```python
from build123d import *
from build123d import SkipClean  # not in build123d's __all__

# Parameters (mm, degrees)
F1_DEPTH  = 25.4
F1_FACE_R = 17.6985452631
F2_DEPTH  = 25.4
F3_DEPTH  = 25.4


with BuildPart() as f1:
    # F0 (on Top) → F1 (new body)
    with BuildSketch(Plane.XY):
        with BuildLine():
            ThreePointArc((0, 41.7947099158), (29.5533227992, 29.5533227992), (41.7947099158, 0))
            ThreePointArc((41.7947099158, 0), (29.5533227992, -29.5533227992), (0, -41.7947099158))
            Line((0, -41.7947099158), (0, -41.9407263398))
            Line((0, -41.9407263398), (115.8670112491, -41.9407263398))
            Line((115.8670112491, -41.9407263398), (115.8670112491, 41.7947099158))
            Line((115.8670112491, 41.7947099158), (0, 41.7947099158))
        make_face()
        with BuildLine():
            ThreePointArc((0, -41.7947099158), (29.5533227992, -29.5533227992), (41.7947099158, 0))
            ThreePointArc((41.7947099158, 0), (29.5533227992, 29.5533227992), (0, 41.7947099158))
            Line((0, 41.7947099158), (0, 17.6985452631))
            ThreePointArc((0, 17.6985452631), (12.5147613727, 12.5147613727), (17.6985452631, 0))
            ThreePointArc((17.6985452631, 0), (12.5147613727, -12.5147613727), (0, -17.6985452631))
            Line((0, -17.6985452631), (0, -41.7947099158))
        make_face()
        with BuildLine():
            Line((0, 17.6985452631), (0, 41.7947099158))
            ThreePointArc((0, 41.7947099158), (-41.7947099158, 0), (0, -41.7947099158))
            Line((0, -41.7947099158), (0, -17.6985452631))
            ThreePointArc((0, -17.6985452631), (-17.6985452631, 0), (0, 17.6985452631))
        make_face()
    extrude(amount=F1_DEPTH)

    # F1_face (on face) + F0 (on Top) → F2 (join)
    with BuildSketch(Plane(origin=(44.792448598, -0.0617990101, 25.4), x_dir=(1, 0, 0), z_dir=(0, 0, 1))):
        with BuildLine():
            Line((71.0745626511, 41.8565089259), (-44.792448598, 41.8565089259))
            ThreePointArc((-44.792448598, 41.8565089259), (-86.5871585138, 0.0617990101), (-44.792448598, -41.7329109057))
            Line((-44.792448598, -41.7329109057), (-44.792448598, -41.8789273297))
            Line((-44.792448598, -41.8789273297), (71.0745626511, -41.8789273297))
            Line((71.0745626511, -41.8789273297), (71.0745626511, 41.8565089259))
        make_face()
        with Locations((-44.792448598, 0.0617990101)):
            Circle(F1_FACE_R, mode=Mode.SUBTRACT)
    with BuildSketch(Plane.XY):
        with BuildLine():
            ThreePointArc((0, -41.7947099158), (29.5533227992, -29.5533227992), (41.7947099158, 0))
            ThreePointArc((41.7947099158, 0), (29.5533227992, 29.5533227992), (0, 41.7947099158))
            Line((0, 41.7947099158), (0, 17.6985452631))
            ThreePointArc((0, 17.6985452631), (12.5147613727, 12.5147613727), (17.6985452631, 0))
            ThreePointArc((17.6985452631, 0), (12.5147613727, -12.5147613727), (0, -17.6985452631))
            Line((0, -17.6985452631), (0, -41.7947099158))
        make_face()
        with BuildLine():
            ThreePointArc((0, 41.7947099158), (29.5533227992, 29.5533227992), (41.7947099158, 0))
            ThreePointArc((41.7947099158, 0), (29.5533227992, -29.5533227992), (0, -41.7947099158))
            Line((0, -41.7947099158), (0, -41.9407263398))
            Line((0, -41.9407263398), (115.8670112491, -41.9407263398))
            Line((115.8670112491, -41.9407263398), (115.8670112491, 41.7947099158))
            Line((115.8670112491, 41.7947099158), (0, 41.7947099158))
        make_face()
        with BuildLine():
            Line((0, 17.6985452631), (0, 41.7947099158))
            ThreePointArc((0, 41.7947099158), (-41.7947099158, 0), (0, -41.7947099158))
            Line((0, -41.7947099158), (0, -17.6985452631))
            ThreePointArc((0, -17.6985452631), (-17.6985452631, 0), (0, 17.6985452631))
        make_face()
    with SkipClean():  # cleaning this boolean's faces spoils the solid; the shape is the same uncleaned
        extrude(amount=F2_DEPTH)

    # F3 (cut): a face of the model
    f3_faces = [f1.faces().sort_by_distance(p)[0] for p in [
        (44.792448598, -0.0617990101, 50.8),
    ]]
    extrude(f3_faces, amount=-F3_DEPTH, mode=Mode.SUBTRACT)


solid = f1.part
```
Source: CAD feature listing. Evaluate the final solid. Frame: model axes, mm. Give positions to 0.01 mm unless a question says otherwise; leave off trailing zeros. Write each loop counter-clockwise with the first axis right and the second up, starting at its lowest first coordinate (ties: lowest second). Pieces come first, ordered by that corner, then holes.
1. Section query B-B (y = 7). Return the cut outline in (x, z), then the cut area to 3 significant figures.
2. First-contact query: pin 1 (2 mm diameter, centred on y = -3, z = 9, fed in from -X); pin 2 (10 mm diameter, centred on x = -20.5, z = 12.5, fed in from -Y); pin 3 (12 mm diameter, centred on x = -12, z = 20.5, fed in from +Y). Flat tips, straight axial feed; report the tip coordinate or a pass-through.
3. Section query C-C (y = 23.5). Return the cut outline in (x, z).
4. Section query A-A (z = 6.5). Return the cut outline in (x, y), then the cut area to 3 significant figures.
5. Section query D-D (y = -23). Return the cut outline in (x, z), then the cut area to 3 significant figures.
6. Material intervals for line 1 along Y through (x, z) = (1, 2.25); line 2 along Y through (x, z) = (9, 2.5); line 3 along X through (y, z) = (16, 8), sorted ascending.
Output values:
1. outline: (-41.2, 0) - (-16.26, 0) - (-16.26, 25.4) - (-41.2, 25.4) - close; (16.26, 0) - (115.87, 0) - (115.87, 25.4) - (16.26, 25.4) - close
1. area: 3,160 mm2
2. pin 1: stops at x = -41.75
2. pin 2: stops at y = -38.81
2. pin 3: stops at y = 41.36
3. outline: (-34.56, 0) - (115.87, 0) - (115.87, 25.4) - (-34.56, 25.4) - close
4. outline: (0, -41.94) - (115.87, -41.94) - (115.87, 41.79) - (0, 41.79) arc R41.79 ccw to (0, -41.79) - close; hole circle Ø35.4 at (0, 0)
4. area: 11,500 mm2
5. outline: (-34.9, 0) - (115.87, 0) - (115.87, 25.4) - (-34.9, 25.4) - close
5. area: 3,830 mm2
6. line 1: y = -41.94 to -17.67, 17.67 to 41.79
6. line 2: y = -41.94 to -15.24, 15.24 to 41.79
6. line 3: x = -38.61 to -7.57, 7.57 to 115.87
